Part model, mm, in its own coordinate system. Face numbers are marked on the shaded views. A direction names the side the tool comes from. Give positions to 0.01 mm unless a question says otherwise; leave off trailing zeros. Write each loop counter-clockwise with the first axis right and the second up, starting at its lowest first coordinate (ties: lowest second). Pieces come first, ordered by that corner, then holes. Notation, with made-up numbers: M 49,85 L 105,85 A29 ccw 105,120 Z; hole C 69,0 d1. An arc over 180 degrees is marked long. Use a Markdown table: item, result.
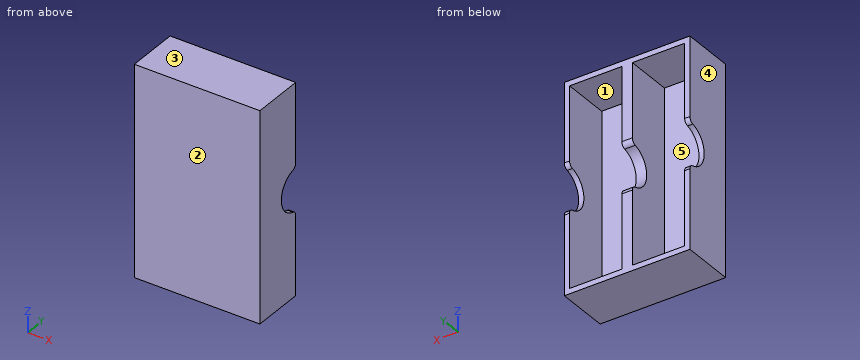
Autodesk Inventor part; units mm, degrees
ref_plane "YZ Plane" through (0, 0, 0) normal (1, 0, 0) x (0, 1, 0)
ref_plane "XZ Plane" through (0, 0, 0) normal (0, 1, 0) x (-1, 0, 0)
ref_plane "XY Plane" through (0, 0, 0) normal (0, 0, 1) x (1, 0, 0)
sketch "Sketch1" plane through (0, 0, 0) normal (0, 1, 0) x (-1, 0, 0)
  line L0 (0, 0) -> (120, 0)
  line L1 (120, 0) -> (120, -200)
  line L2 (120, -200) -> (0, -200)
  line L3 (0, -200) -> (0, 0)
  dimension "d0" = 120
  dimension "d1" = 200
extrude "Extrusion1" add sketch "Sketch1" along normal blind 50
sketch "Sketch2" plane through (0, 50, 0) normal (0, 1, 0) x (1, 0, 0)
  line L0 (-5, 5) -> (-5, 195)
  line L1 (0, 200) -> (-120, 200)
  line L2 (-5, 195) -> (-55, 195)
  line L3 (-55, 195) -> (-55, 5)
  line L4 (-55, 5) -> (-5, 5)
  line L5 (-115, 5) -> (-65, 5)
  line L6 (-65, 5) -> (-65, 195)
  line L7 (-65, 195) -> (-115, 195)
  line L8 (-115, 195) -> (-115, 5)
  point P0 (0, 0)
  dimension "d4" = 190
  dimension "d5" = 50
  dimension "d6" = 50
  dimension "d7" = 190
extrude "Extrusion2" cut sketch "Sketch2" against normal blind 45
sketch "Sketch4" plane through (0, 0, 0) normal (1, 0, 0) x (0, 0, -1)
  line L0 (5, 50) -> (195, 50)
  circle A0 centre (100, 50) radius 20
  point P0 (0, 0)
  dimension "d10" = 40
extrude "Extrusion3" cut sketch "Sketch4" against normal blind 120
fillet "Fillet1" radius 5 6 edges at (-117.5, 50, -120) (-117.5, 50, -80) (-60, 50, -120) (-60, 50, -80) (-2.5, 50, -120) (-2.5, 50, -80)
properties part number "Box"
1. Two-plate mould, pull along Z, no slides. Class the marked faces 1, 2 and 3: released by +Z, released by -Z, zero draft, split by the parting line, or undercut.
Findings below:
| item | result |
|---|---|
| face 1 | undercut |
| face 2 | zero draft |
| face 3 | released by +Z |
2. Drop a flat-ended pin along its axis: P1, Ø6, axis at x = -101.5, z = -69, coming from the +Y side. Give the stop position or say it passes through.
Findings below:
| item | result |
|---|---|
| P1 | y = 5 |
3. Tool access for the marked faces 4 and 5: list every direction of +Z, -Z, +X, -X, +Y, -Y with a clear straight run to the whole face (end or side of a thin tool).
Findings below:
| item | result |
|---|---|
| face 4 | +Z, -Z, -X, +Y, -Y |
| face 5 | +Y |
4. Cut at A-A, the plane y = 23. Give the cut face in (x, z), then the cut area to 3 significant figures.
Findings below:
| item | result |
|---|---|
| outline | M -120,-200 L 0,-200 L 0,0 L -120,0 Z; hole M -115,-195 L -65,-195 L -65,-5 L -115,-5 Z; hole M -55,-195 L -5,-195 L -5,-5 L -55,-5 Z |
| area | 5,000 mm2 |
5. Drill centre lines: L1, parallel to X at y = 8, z = -98; L2, parallel to Z at x = -96.5, y = 41.5; L3, parallel to Y at x = -66, z = -139. Where is each one in solid material? Low to high.
Findings below:
| item | result |
|---|---|
| L1 | -120 to -115, -65 to -55, -5 to 0 |
| L2 | -200 to -195, -5 to 0 |
| L3 | 0 to 5 |
6. Cut at D-D, the plane z = -15.5. Give the cut face in (x, y), then the cut area to 3 significant figures.
Findings below:
| item | result |
|---|---|
| outline | M -120,0 L 0,0 L 0,50 L -5,50 L -5,5 L -55,5 L -55,50 L -65,50 L -65,5 L -115,5 L -115,50 L -120,50 Z |
| area | 1,500 mm2 |
7. Cut at B-B, the plane y = 42. Give the cut face in (x, z).
Findings below:
| item | result |
|---|---|
| outline | M -120,-200 L 0,-200 L 0,-118.33 L -5,-118.33 L -5,-195 L -55,-195 L -55,-118.33 L -65,-118.33 L -65,-195 L -115,-195 L -115,-118.33 L -120,-118.33 Z; M -120,-81.67 L -115,-81.67 L -115,-5 L -65,-5 L -65,-81.67 L -55,-81.67 L -55,-5 L -5,-5 L -5,-81.67 L 0,-81.67 L 0,0 L -120,0 Z |
8. Cut at C-C, the plane x = -112. Give the cut face in (y, z).
Findings below:
| item | result |
|---|---|
| outline | M 0,-200 L 50,-200 L 50,-195 L 5,-195 L 5,-5 L 50,-5 L 50,0 L 0,0 Z |
